For this review, use the dimensioned drawing (mm, ordinates from the lowest corner) and the shaded views. A direction names the side the tool comes from. Coordinates: 2 decimals unless noted, no trailing zeros. Loops run counter-clockwise (first coordinate to the right, second up) from the corner with the lowest first, then second, coordinate; pieces in that order, holes last. Notation, with made-up numbers: (-9.5, -26.5) - (30.5, -26.5) arc R34 cw to (30.5, 11.5) - close; hole circle Ø8 at (-29, 82.5). An arc over 180 degrees is marked (long way). Use a Markdown table: item, result. Add a question column.
1) Add section D-D, the plane y = 11. Give the boundary of the cut face in (x, z).
2) Add section B-B, the plane x = 30. Give the boundary of the cut face in (y, z).
3) Add section A-A, the plane y = 32. Give the boundary of the cut face in (x, z).
4) Clearance check with flat-ended pins moving along their axes: pin 1 (1 mm diameter, centred on x = 30, y = 34.5, fed in from +Z); pin 2 (3 mm diameter, centred on y = 49.5, z = 43, fed in from +X); pin 3 (22 mm diameter, centred on x = 55, y = 52.5, fed in from +Z). State where each tip first meets the part, or that it passes through.
5) Add section C-C, the plane z = 12. Give the boundary of the cut face in (x, y), and give its area (3 significant figures).
6) For the marked faces 1, 2 and 3, list the 3-axis set-ups (+Z, -Z, +X, -X, +Y, -Y) from which the entire face can be reached by the end or side of a thin tool; tool diameter is ignored.
7) To check wall thickness, follow L1, parallel to Z at x = 46, y = 34; L2, parallel to X at y = 50, z = 42.5; L3, parallel to Y at x = 48.5, z = 33.5. State the ranges of each line that lie inside material, in increasing order. Write a range as [from, to].
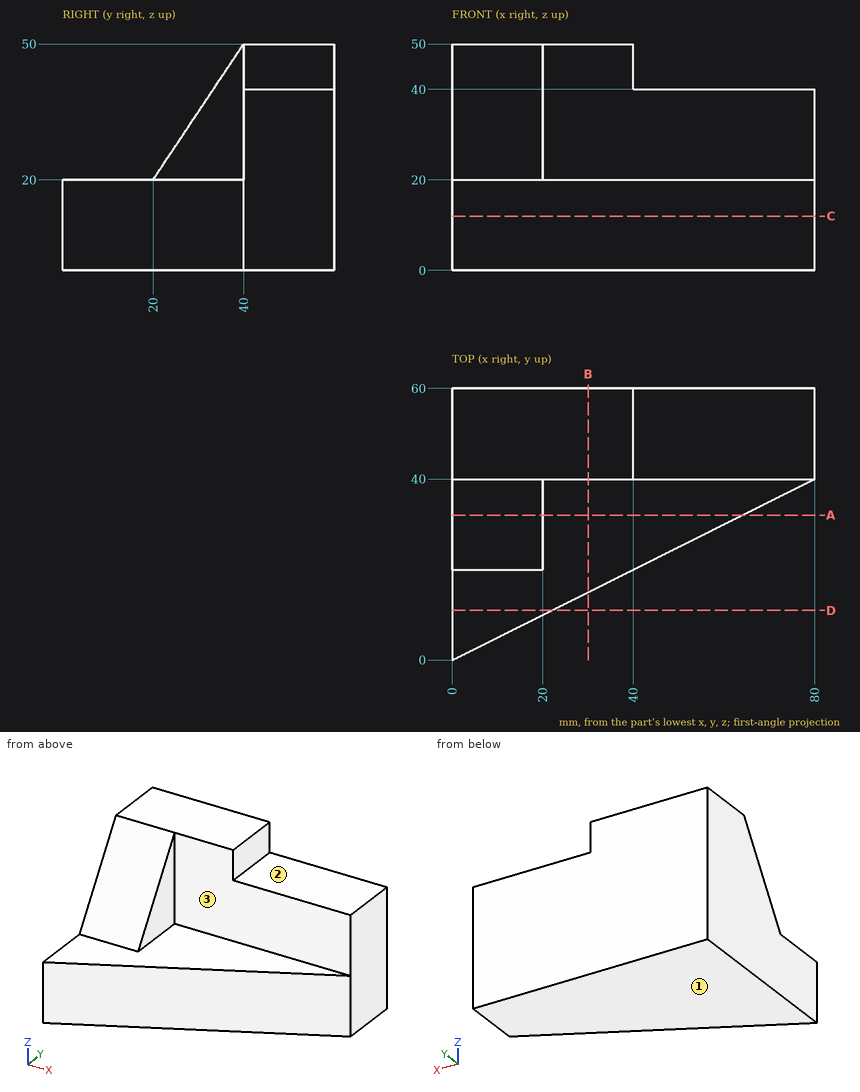
From the geometry:
| question | item | result |
|---|---|---|
| 1 | outline | (0, 0) - (22, 0) - (22, 20) - (0, 20) - close |
| 2 | outline | (15, 0) - (60, 0) - (60, 50) - (40, 50) - (40, 20) - (15, 20) - close |
| 3 | outline | (0, 0) - (64, 0) - (64, 20) - (20, 20) - (20, 38) - (0, 38) - close |
| 4 | pin 1 | stops at z = 20 |
| 4 | pin 2 | stops at x = 40 |
| 4 | pin 3 | stops at z = 40 |
| 5 | outline | (0, 0) - (80, 40) - (80, 60) - (0, 60) - close |
| 5 | area | 3,200 mm^2 |
| 6 | face 1 | -Z, +X, -X, +Y, -Y |
| 6 | face 2 | +Z, +X, +Y, -Y |
| 6 | face 3 | +Z, +X, -Y |
| 7 | L1 | z = [0, 20] |
| 7 | L2 | x = [0, 40] |
| 7 | L3 | y = [40, 60] |
